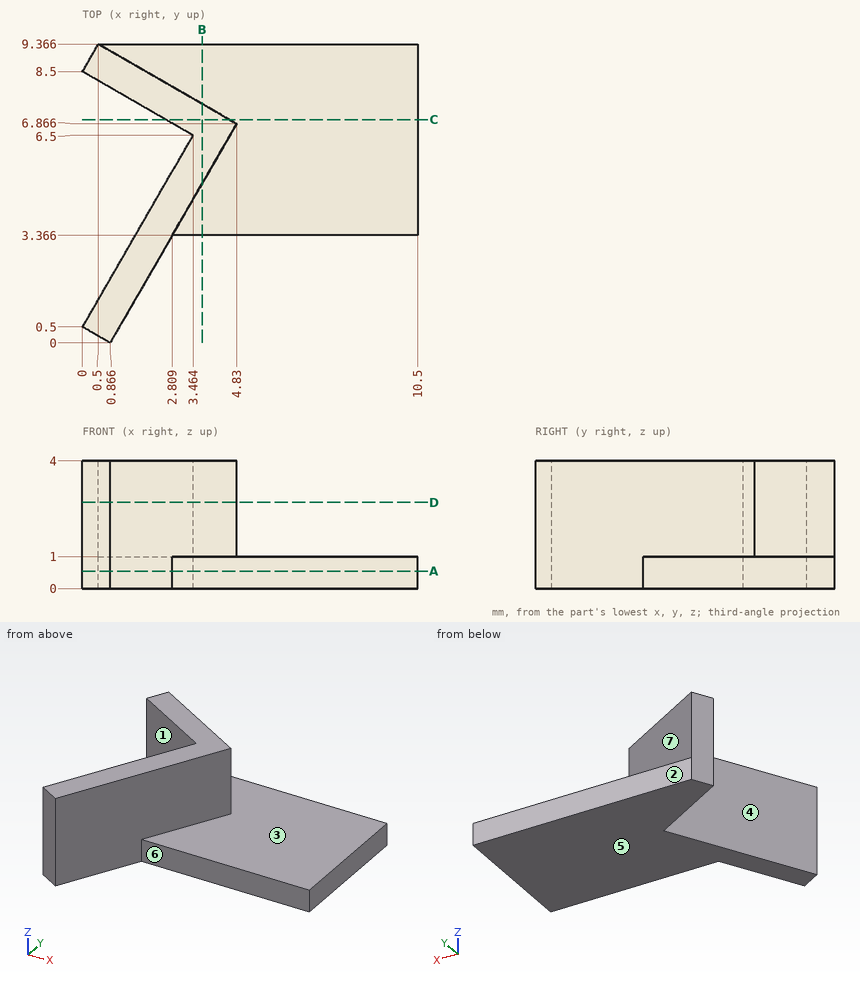
Here's the drawing with two shaded views (mm, measured from the low corner). I have some questions. A direction names the side the tool comes from. Coordinates: 2 decimals unless noted, no trailing zeros. Write each loop counter-clockwise with the first axis right and the second up, starting at its lowest first coordinate (ties: lowest second). Pieces come first, ordered by that corner, then holes.
Item 1: Will these pins go through, and if not, where does the flat tip stop? pin 1 (5 mm diameter, centred on x = 5.5, y = 3.5, fed in from +Z); pin 2 (1.5 mm diameter, centred on y = 1.5, z = 0.5, fed in from -X) (1 decimal).
Item 2: I want a section at D-D on z = 2.7. Write out the boundary of the cut face in (x, y), and give its area (3 significant figures).
Item 3: I want a section at B-B on x = 3.75. Write out the boundary of the cut face in (y, z) (1 decimal), and give its area (3 significant figures).
Item 4: I want a section at A-A on z = 0.55. Write out the boundary of the cut face in (x, y).
Item 5: On a 3-axis mill with a long thin cutter (end or side, diameter ignored), from which of +Z, -Z, +X, -X, +Y, -Y can I reach the whole of each face in a straight line? I mean the marked faces 5, 6 and 7. Say none if no direction works.
Item 6: If we mould it in two halves opening along Y, with no side actions, what happens to the marked faces 1, 2, 3 and 4? For each: +Y half, -Y half, draft (parallel to the pull), parting line (faces both ways), or undercut.
Item 7: I want a section at C-C on y = 7. Write out the boundary of the cut face in (x, z).
Item 8: If I drill on line 1 (Y direction, x = 1.5, z = 3.5) (1 decimal); line 2 (Z direction, x = 5, y = 8); line 3 (Y direction, x = 3, z = 2.9) (1 decimal), over which ranges is the centre line in solid material (lowest first)?
Findings below:
1. pin 1: stops at z = 4
1. pin 2: stops at x = 0.1
2. outline: (0, 0.5) - (0.87, 0) - (4.83, 6.87) - (0.5, 9.37) - (0, 8.5) - (3.46, 6.5) - close
2. area: 11.9 mm2
3. outline: (3.4, 0) - (9.4, 0) - (9.4, 1) - (7.5, 1) - (7.5, 4) - (5, 4) - (5, 1) - (3.4, 1) - close
3. area: 13.5 mm2
4. outline: (0, 0.5) - (0.87, 0) - (2.81, 3.37) - (10.5, 3.37) - (10.5, 9.37) - (0.5, 9.37) - (0, 8.5) - (3.46, 6.5) - close
5. face 5: -Z, +X, -X, +Y, -Y
5. face 6: +Z, -Z, +X, -Y
5. face 7: +Z, +X, +Y
6. face 1: undercut
6. face 2: +Y half
6. face 3: draft
6. face 4: undercut
7. outline: (2.6, 0) - (10.5, 0) - (10.5, 1) - (4.6, 1) - (4.6, 4) - (2.6, 4) - close
8. line 1: y = 1.1 to 3.1, 7.6 to 8.8
8. line 2: z = 0 to 1
8. line 3: y = 3.7 to 5.7, 6.8 to 7.9
